Model file for the job. Use its own axes, mm. Face numbers are marked on the shaded views. Coordinates: 2 decimals unless noted, no trailing zeros. Write each loop counter-clockwise with the first axis right and the second up, starting at its lowest first coordinate (ties: lowest second). Pieces come first, ordered by that corner, then holes. Notation, with made-up numbers: (18.5, 1) - (52.5, 1) arc R34 cw to (52.5, 37) - close; hole circle Ø4 at (55, 59.5). An arc over 180 degrees is marked (long way). Put each result on its own line as item: value. Start each with the question number.
1. Drop flat-ended pins along their axis: P1, Ø1.1, axis at y = 2.5, z = 0.5, coming from the -X side; P2, Ø2.5, axis at y = -1, z = 0.5, coming from the +X side; P3, Ø3, axis at x = -4.5, z = 4.5, coming from the +Y side. Give the stop position or say it passes through.
2. Saw through at A-A, the plane y = -1. Write the cut outline in (x, z).
3. Saw through at C-C, the plane z = 8.25. Write the cut outline in (x, y), plus the area to 3 significant figures.
4. Pull direction Z, two halves, no side cores. Call the marked faces 1, 2 and 3: released by +Z, released by -Z, zero draft, split by the parting line, or undercut.
5. Drill centre lines: L1, parallel to Z at x = 9, y = -14; L2, parallel to Y at x = 7, z = 1; L3, parallel to Z at x = 7, y = 2. Where is each one in solid material? Low to high. Write a range as from..to.
6. Saw through at D-D, the plane y = 17. Write the cut outline in (x, z), plus the area to 3 significant figures.
7. Saw through at B-B, the plane x = 1. Write the cut outline in (y, z).
```python
from build123d import *

# Parameters (mm, degrees)
F1_DEPTH     = 20
F2_DEPTH     = 13
F0_W         = 13
F0_H         = 2.1210866805
F3_R         = 5
F4_R         = 5
F6_DEPTH     = 8
F7_R         = 5
F8_T1_DEPTH  = 12
F8_T3_DEPTH  = 16
F8_T6_ANGLE  = 90
F8_T8_ANGLE  = 90
F8_T10_ANGLE = 90
F8_T12_ANGLE = 90


# Not quite as in the source:
# - a fillet or chamfer that OpenCascade refuses, or shapes differently, is made with other operations: its cross-section is extruded or revolved along the edge and cut away or added


with BuildPart() as f1:
    # F0 (on Front) → F1 (new body, symmetric)
    with BuildSketch(Plane.XZ):
        Polygon((0, 13.6210866805), (0, 15), (-25, 15), (-25, 13.6210866805), (-11, 13.6210866805), align=None)
        Polygon((25, 15), (0, 15), (0, 13.6210866805), (11, 13.6210866805), (25, 13.6210866805), align=None)
    extrude(amount=F1_DEPTH, both=True)

    # F0 (on Front) → F2 (join, symmetric)
    with BuildSketch(Plane.XZ):
        Polygon((0, 12.1210866805), (0, 13.6210866805), (-11, 13.6210866805), (-11, 12.1210866805), (-6.4361323602, 12.1210866805), align=None)
        Polygon((11, 13.6210866805), (0, 13.6210866805), (0, 12.1210866805), (6.4361323602, 12.1210866805), (11, 12.1210866805), align=None)
    extrude(amount=F2_DEPTH, both=True)

    # F4
    f4_edges = [f1.edges().sort_by_distance(p)[0] for p in [
        (-25, -20, 14.310543),
        (-25, 20, 14.310543),
        (25, -20, 14.310543),
        (25, 20, 14.310543),
    ]]
    fillet(f4_edges, radius=F4_R)

    # F0 (on Front) → F6 (join, symmetric)
    with BuildSketch(Plane.XZ):
        with BuildLine():
            Line((0, 2.1210866805), (0, 12.1210866805))
            Line((0, 12.1210866805), (-6.4361323602, 12.1210866805))
            ThreePointArc((-6.4361323602, 12.1210866805), (-9.1727786789, 6.7631671822), (-13, 2.1210866805))
            Line((-13, 2.1210866805), (0, 2.1210866805))
        make_face()
        with Locations((-6.5, 1.0605433403)):
            Rectangle(F0_W, F0_H)
        with BuildLine():
            Line((6.4361323602, 12.1210866805), (0, 12.1210866805))
            Line((0, 12.1210866805), (0, 2.1210866805))
            Line((0, 2.1210866805), (13, 2.1210866805))
            ThreePointArc((13, 2.1210866805), (9.1727786789, 6.7631671822), (6.4361323602, 12.1210866805))
        make_face()
        with Locations((6.5, 1.0605433403)):
            Rectangle(F0_W, F0_H)
    extrude(amount=F6_DEPTH, both=True)

    # F7
    f7_edges = [f1.edges().sort_by_distance(p)[0] for p in [
        (-11, -13, 12.871087),
        (-11, 13, 12.871087),
        (11, -13, 12.871087),
        (11, 13, 12.871087),
    ]]
    fillet(f7_edges, radius=F7_R)

    # F8: fillet of radius 5 on 1 edges, made by hand

    # F8_s2 → F8_t1 (cut)
    with BuildSketch(Plane.YZ.offset(-6)):
        with BuildLine():
            ThreePointArc((-13, 13.6210866805), (-11.3657774588, 12.5113144519), (-9.4292857857, 12.1210866805))
            Line((-9.4292857857, 12.1210866805), (-9.4292857857, 12.0210866805))
            Line((-9.4292857857, 12.0210866805), (-13, 12.0210866805))
            Line((-13, 12.0210866805), (-13.1, 12.1210866805))
            ThreePointArc((-13.1, 12.1210866805), (-13.1, 12.8710866805), (-13.0714142843, 13.5510866805))
            Line((-13.0714142843, 13.5510866805), (-13, 13.6210866805))
        make_face()
        with BuildLine():
            ThreePointArc((13, 13.6210866805), (11.3657774588, 12.5113144519), (9.4292857857, 12.1210866805))
            Line((9.4292857857, 12.1210866805), (9.4292857857, 12.0210866805))
            Line((9.4292857857, 12.0210866805), (13, 12.0210866805))
            Line((13, 12.0210866805), (13.1, 12.1210866805))
            ThreePointArc((13.1, 12.1210866805), (13.1, 12.8710866805), (13.0714142843, 13.5510866805))
            Line((13.0714142843, 13.5510866805), (13, 13.6210866805))
        make_face()
    extrude(amount=F8_T1_DEPTH, mode=Mode.SUBTRACT)

    # F8_s4 → F8_t3 (cut)
    with BuildSketch(Plane.XZ.offset(-8)):
        with BuildLine():
            ThreePointArc((11, 13.6210866805), (9.3657774588, 12.5113144519), (7.4292857857, 12.1210866805))
            Line((7.4292857857, 12.1210866805), (7.4292857857, 12.0210866805))
            Line((7.4292857857, 12.0210866805), (11, 12.0210866805))
            Line((11, 12.0210866805), (11.1, 12.1210866805))
            ThreePointArc((11.1, 12.1210866805), (11.1, 12.8710866805), (11.0714142843, 13.5510866805))
            Line((11.0714142843, 13.5510866805), (11, 13.6210866805))
        make_face()
        with BuildLine():
            ThreePointArc((-11, 13.6210866805), (-9.3657774588, 12.5113144519), (-7.4292857857, 12.1210866805))
            Line((-7.4292857857, 12.1210866805), (-7.4292857857, 12.0210866805))
            Line((-7.4292857857, 12.0210866805), (-11, 12.0210866805))
            Line((-11, 12.0210866805), (-11.1, 12.1210866805))
            ThreePointArc((-11.1, 12.1210866805), (-11.1, 12.8710866805), (-11.0714142843, 13.5510866805))
            Line((-11.0714142843, 13.5510866805), (-11, 13.6210866805))
        make_face()
    extrude(amount=F8_T3_DEPTH, mode=Mode.SUBTRACT)

    # F8_s5 → F8_t6 (revolve, cut)
    with BuildSketch(Plane.XZ.offset(8)):
        with BuildLine():
            ThreePointArc((-11, 13.6210866805), (-9.3657774588, 12.5113144519), (-7.4292857857, 12.1210866805))
            Line((-7.4292857857, 12.1210866805), (-7.4292857857, 12.0210866805))
            Line((-7.4292857857, 12.0210866805), (-11, 12.0210866805))
            Line((-11, 12.0210866805), (-11.1, 12.1210866805))
            ThreePointArc((-11.1, 12.1210866805), (-11.1, 12.8710866805), (-11.0714142843, 13.5510866805))
            Line((-11.0714142843, 13.5510866805), (-11, 13.6210866805))
        make_face()
    revolve(axis=Axis((-6, -8, 12.1210866805), (0, 0, 1)), revolution_arc=F8_T6_ANGLE, mode=Mode.SUBTRACT)

    # F8_s7 → F8_t8 (revolve, cut)
    with BuildSketch(Plane.XZ.offset(8)):
        with BuildLine():
            ThreePointArc((11, 13.6210866805), (9.3657774588, 12.5113144519), (7.4292857857, 12.1210866805))
            Line((7.4292857857, 12.1210866805), (7.4292857857, 12.0210866805))
            Line((7.4292857857, 12.0210866805), (11, 12.0210866805))
            Line((11, 12.0210866805), (11.1, 12.1210866805))
            ThreePointArc((11.1, 12.1210866805), (11.1, 12.8710866805), (11.0714142843, 13.5510866805))
            Line((11.0714142843, 13.5510866805), (11, 13.6210866805))
        make_face()
    revolve(axis=Axis((6, -8, 12.1210866805), (0, 0, -1)), revolution_arc=F8_T8_ANGLE, mode=Mode.SUBTRACT)

    # F8_s9 → F8_t10 (revolve, cut)
    with BuildSketch(Plane.YZ.offset(6)):
        with BuildLine():
            ThreePointArc((13, 13.6210866805), (11.3657774588, 12.5113144519), (9.4292857857, 12.1210866805))
            Line((9.4292857857, 12.1210866805), (9.4292857857, 12.0210866805))
            Line((9.4292857857, 12.0210866805), (13, 12.0210866805))
            Line((13, 12.0210866805), (13.1, 12.1210866805))
            ThreePointArc((13.1, 12.1210866805), (13.1, 12.8710866805), (13.0714142843, 13.5510866805))
            Line((13.0714142843, 13.5510866805), (13, 13.6210866805))
        make_face()
    revolve(axis=Axis((6, 8, 12.1210866805), (0, 0, -1)), revolution_arc=F8_T10_ANGLE, mode=Mode.SUBTRACT)

    # F8_s11 → F8_t12 (revolve, cut)
    with BuildSketch(Plane.XZ.offset(-8)):
        with BuildLine():
            ThreePointArc((-11, 13.6210866805), (-9.3657774588, 12.5113144519), (-7.4292857857, 12.1210866805))
            Line((-7.4292857857, 12.1210866805), (-7.4292857857, 12.0210866805))
            Line((-7.4292857857, 12.0210866805), (-11, 12.0210866805))
            Line((-11, 12.0210866805), (-11.1, 12.1210866805))
            ThreePointArc((-11.1, 12.1210866805), (-11.1, 12.8710866805), (-11.0714142843, 13.5510866805))
            Line((-11.0714142843, 13.5510866805), (-11, 13.6210866805))
        make_face()
    revolve(axis=Axis((-6, 8, 12.1210866805), (0, 0, -1)), revolution_arc=F8_T12_ANGLE, mode=Mode.SUBTRACT)


with BuildPart() as f2:
    # F0 (on Front) → F2, piece 2 (new body, symmetric)
    with BuildSketch(Plane.XZ):
        with Locations((-6.5, 1.0605433403)):
            Rectangle(F0_W, F0_H)
        with Locations((6.5, 1.0605433403)):
            Rectangle(F0_W, F0_H)
    extrude(amount=F2_DEPTH, both=True)

    # F3
    f3_edges = [f2.edges().sort_by_distance(p)[0] for p in [
        (-13, 13, 1.060543),
        (-13, -13, 1.060543),
        (13, -13, 1.060543),
        (13, 13, 1.060543),
    ]]
    fillet(f3_edges, radius=F3_R)


solid = f1.part
```
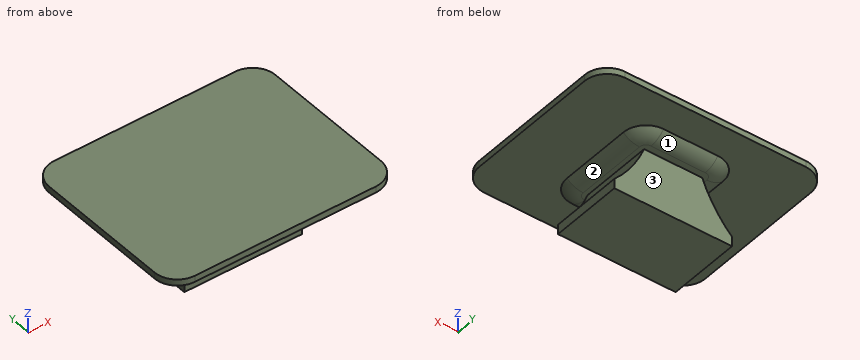
Final values:
1. P1: stops at x = -13
1. P2: stops at x = 13
1. P3: stops at y = 8
2. outline: (-25, 13.62) - (-11, 13.62) arc R5 ccw to (-7.43, 12.12) - (-6.44, 12.12) arc R27.75 cw to (-13, 2.12) - (-13, 0) - (13, 0) - (13, 2.12) arc R27.75 cw to (6.44, 12.12) - (7.43, 12.12) arc R5 ccw to (11, 13.62) - (25, 13.62) - (25, 15) - (-25, 15) - close
3. outline: (-8.26, -8) - (8.26, -8) - (8.26, 8) - (-8.26, 8) - close
3. area: 264 mm²
4. face 1: released by -Z
4. face 2: undercut
4. face 3: zero draft
5. L1: z = 13.62..15
5. L2: y = -8..8
5. L3: z = 0..10.75, 12.12..15
6. outline: (-24.58, 13.62) - (24.58, 13.62) - (24.58, 15) - (-24.58, 15) - close
6. area: 67.8 mm²
7. outline: (-20, 13.62) - (-13, 13.62) arc R5 ccw to (-9.43, 12.12) - (-8, 12.12) - (-8, 0) - (8, 0) - (8, 12.12) - (9.43, 12.12) arc R5 ccw to (13, 13.62) - (20, 13.62) - (20, 15) - (-20, 15) - close
